Autodesk Inventor part; units mm, degrees
ref_plane "YZ Plane" through (0, 0, 0) normal (1, 0, 0) x (0, 1, 0)
ref_plane "XZ Plane" through (0, 0, 0) normal (0, 1, 0) x (-1, 0, 0)
ref_plane "XY Plane" through (0, 0, 0) normal (0, 0, 1) x (1, 0, 0)
sketch "Sketch1" plane through (0, 0, 0) normal (1, 0, 0) x (0, 1, 0)
  line L0 (53.34, 0) -> (53.34, -68.58)
  line L1 (53.34, -68.58) -> (0, -68.58)
  line L2 (0, -68.58) -> (0, 0)
  line L3 (53.34, 0) -> (44.45, 0)
  line L4 (44.45, 0) -> (44.45, 6.858)
  line L5 (44.45, 6.858) -> (32.004, 6.858)
  line L6 (32.004, 6.858) -> (32.004, 0)
  line L7 (44.45, 0) -> (53.34, 0)
  line L8 (0, 0) -> (3.6068, 0)
  line L9 (3.6068, 0) -> (3.6068, 1.524)
  line L10 (3.6068, 1.524) -> (12.4968, 1.524)
  line L11 (12.4968, 1.524) -> (12.4968, 0)
  line L12 (0, 0) -> (3.6068, 0)
  line L13 (12.4968, 0) -> (32.004, 0)
  dimension "d0" = 53.34
  dimension "d1" = 68.58
  dimension "d2" = 8.89
  dimension "d3" = 6.858
  dimension "d4" = 12.446
  dimension "d5" = 3.6068
  dimension "d6" = 1.524
  dimension "d7" = 8.89
extrude "Extrusion1" add sketch "Sketch1" along normal blind 10.922
properties part number "msheehan_uno_board"
Source: CAD feature listing. Evaluate the final solid. Frame: model axes, mm. A direction names the side the tool comes from. Round coordinates to 2 decimals unless told otherwise and drop trailing zeros. Loops run counter-clockwise (first coordinate to the right, second up) from the corner with the lowest first, then second, coordinate; pieces in that order, holes last. Notation, with made-up numbers: M 6.5,86.25 L 46.5,86.25 A21 ccw 46.5,103.25 Z; hole C 34.5,39.5 d5. An arc over 180 degrees is marked long. Return JSON: item names as keys, results as strings. Group by question number.
1. Section query C-C on y = 22.5. Output: boundary loops of the cut face in (x, z), and give its area (3 significant figures).
2. Mould query, pull axis Y, two halves, no side actions, for faces 6 (the face through (5, 8, 1.524)), 7 (the face through (5, 22, 0)), 8 (the face through (5, 3.607, 1)). Classes: released by +Y, released by -Y, zero draft, split by the parting line, or undercut.
3. Section query A-A on x = 2. Output: boundary loops of the cut face in (y, z).
4. Section query B-B on y = 5. Output: boundary loops of the cut face in (x, z).
5. Pin query (flat end, axial travel): pin 1 (4 mm diameter, centred on x = 6.5, y = 1, fed in from +Z); pin 2 (0.5 mm diameter, centred on x = 3, z = 1, fed in from -Y); pin 3 (5.5 mm diameter, centred on x = 7.5, z = 4.5, fed in from -Y). Return the tip coordinate at first contact, or that it passes through.
6. Material intervals for line 1 along Z through (x, y) = (8, 48.5); line 2 along Z through (x, y) = (3, 8.5); line 3 along Y through (x, z) = (5, 2.5), sorted ascending. Write a range as from..to.
7. Reachability of faces 1 (the face through (5, 32.004, 3)), 2 (the face through (5, 2, 0)), 3 (the face through (0, 26, -30)), 4 (the face through (5, 0, -35)), 5 (the face through (5, 49, 0)) from +Z, -Z, +X, -X, +Y, -Y: full face, straight path, thin tool, end or side. Return the list, or none.
Checks:
{
 "1": {"outline": "M 0,-68.58 L 10.92,-68.58 L 10.92,0 L 0,0 Z", "area": "749 mm²"},
 "2": {"face 6": "zero draft", "face 7": "undercut", "face 8": "released by -Y"},
 "3": {"outline": "M 0,-68.58 L 53.34,-68.58 L 53.34,0 L 44.45,0 L 44.45,6.86 L 32,6.86 L 32,0 L 12.5,0 L 12.5,1.52 L 3.61,1.52 L 3.61,0 L 0,0 Z"},
 "4": {"outline": "M 0,-68.58 L 10.92,-68.58 L 10.92,1.52 L 0,1.52 Z"},
 "5": {"pin 1": "stops at z = 0", "pin 2": "stops at y = 3.61", "pin 3": "stops at y = 32"},
 "6": {"line 1": "z = -68.58..0", "line 2": "z = -68.58..1.52", "line 3": "y = 32..44.45"},
 "7": {"face 1": "+Z, +X, -X", "face 2": "+Z, +X, -X, -Y", "face 3": "+Z, -Z, -X, +Y, -Y", "face 4": "+Z, -Z, +X, -X, -Y", "face 5": "+Z, +X, -X, +Y"}
}
